```python
from build123d import *

# Parameters (mm, degrees)
F1_DEPTH = 50


with BuildPart() as f1:
    # F0 (on Right) → F1 (new body)
    with BuildSketch(Plane.YZ):
        with BuildLine():
            Line((-33.1, -0.25), (-33.35, -0.25))
            Line((-33.35, -0.25), (-33.35, 0))
            Line((-33.35, 0), (-33.35, 50.8))
            Line((-33.35, 50.8), (-33.35, 51.05))
            Line((-33.35, 51.05), (-33.1, 51.05))
            Line((-33.1, 51.05), (-31.35, 51.05))
            ThreePointArc((-31.35, 51.05), (-30.642893, 51.342893), (-30.35, 52.05))
            ThreePointArc((-30.35, 52.05), (-30.642893, 52.757107), (-31.35, 53.05))
            Line((-31.35, 53.05), (-33.1, 53.05))
            ThreePointArc((-33.1, 53.05), (-34.69099, 52.39099), (-35.35, 50.8))
            Line((-35.35, 50.8), (-35.35, 0))
            ThreePointArc((-35.35, 0), (-33.885534, -3.535534), (-30.35, -5))
            Line((-30.35, -5), (25.4, -5))
            ThreePointArc((25.4, -5), (28.935534, -3.535534), (30.4, 0))
            Line((30.4, 0), (30.4, 14))
            ThreePointArc((30.4, 14), (30.107107, 14.707107), (29.4, 15))
            ThreePointArc((29.4, 15), (28.692893, 14.707107), (28.4, 14))
            Line((28.4, 14), (28.4, 0))
            Line((28.4, 0), (28.4, -3))
            Line((28.4, -3), (25.4, -3))
            Line((25.4, -3), (0, -3))
            Line((0, -3), (-3, -3))
            Line((-3, -3), (-3, 0))
            Line((-3, 0), (-3, 48.35))
            ThreePointArc((-3, 48.35), (-4.376598, 51.673402), (-7.7, 53.05))
            Line((-7.7, 53.05), (-9.45, 53.05))
            ThreePointArc((-9.45, 53.05), (-10.157107, 52.757107), (-10.45, 52.05))
            ThreePointArc((-10.45, 52.05), (-10.157107, 51.342893), (-9.45, 51.05))
            Line((-9.45, 51.05), (-7.7, 51.05))
            Line((-7.7, 51.05), (-7.45, 51.05))
            Line((-7.45, 51.05), (-7.45, 50.8))
            Line((-7.45, 50.8), (-7.45, 0))
            Line((-7.45, 0), (-7.45, -0.25))
            Line((-7.45, -0.25), (-7.7, -0.25))
            Line((-7.7, -0.25), (-33.1, -0.25))
        make_face()
        with BuildLine():
            Line((-33.35, 51.05), (-33.35, 50.8))
            ThreePointArc((-33.35, 50.8), (-33.276777, 50.976777), (-33.1, 51.05))
            Line((-33.1, 51.05), (-33.35, 51.05))
        make_face()
        with BuildLine():
            ThreePointArc((-7.7, 51.05), (-7.523223, 50.976777), (-7.45, 50.8))
            Line((-7.45, 50.8), (-7.45, 51.05))
            Line((-7.45, 51.05), (-7.7, 51.05))
        make_face()
        with BuildLine():
            ThreePointArc((0, -3), (-2.12132, -2.12132), (-3, 0))
            Line((-3, 0), (-3, -3))
            Line((-3, -3), (0, -3))
        make_face()
        with BuildLine():
            ThreePointArc((-7.45, 0), (-7.523223, -0.176777), (-7.7, -0.25))
            Line((-7.7, -0.25), (-7.45, -0.25))
            Line((-7.45, -0.25), (-7.45, 0))
        make_face()
        with BuildLine():
            Line((-33.35, 0), (-33.35, -0.25))
            Line((-33.35, -0.25), (-33.1, -0.25))
            ThreePointArc((-33.1, -0.25), (-33.276777, -0.176777), (-33.35, 0))
        make_face()
        with BuildLine():
            ThreePointArc((28.4, 0), (27.52132, -2.12132), (25.4, -3))
            Line((25.4, -3), (28.4, -3))
            Line((28.4, -3), (28.4, 0))
        make_face()
    extrude(amount=-F1_DEPTH)


solid = f1.part
```
Work out the finished part from the listing and answer in its coordinate system (mm). A direction names the side the tool comes from. Give positions to 0.01 mm unless a question says otherwise; leave off trailing zeros. Order: outer loops, then holes, each group sorted by start corner. A loop starts at its lowest first (then second) coordinate and runs counter-clockwise, first axis right, second up. Notation, with made-up numbers: (85, 6) - (117, 6) arc R17 cw to (117, 14) - close; hole circle Ø11 at (-26.5, -5.5). An arc over 180 degrees is marked (long way). One line per item, written item: value. Start each with the question number.
1. Consider line 1 (Y direction, x = -16, z = 2.5); line 2 (Y direction, x = -24.5, z = 39.5); line 3 (Z direction, x = -16.5, y = 19.5). Determine where each line is inside the solid, lowest interval first.
2. Section A-A, the plane z = 19 is taken. Write down the section's boundary in (x, y).
3. Each of these flat-tipped pins is pushed along its axis until it touches: pin 1 Ø0.5 at (x, y) = (-29.5, -32) entering from -Z; pin 2 Ø4 at (x, y) = (-44.5, 12.5) entering from +Z; pin 3 Ø1.5 at (x, z) = (-20.5, 46) entering from +Y. Where does it stop, or does it pass through?
4. Which of the six approach directions +Z, -Z, +X, -X, +Y, -Y give full straight-line access (tool end or side, diameter ignored) to faces 1 (the face through (-50, -5, 16)), 2 (the face through (-25, 28.4, 7)), 3 (the face through (-25, -20, -0.25))?
5. For a pull along Y with two mould halves and no side action, classify faces 4 (the face through (-25, -32, 51.05)), 5 (the face through (-25, -35.35, 26)), 6 (the face through (-24.65, -4.34, 51.637)), 7 (the face through (-25, -9, 51.05)) as released by +Y, released by -Y, zero draft, split by the parting line, or undercut.
6. Section B-B, the plane z = 10 is taken. Write down the section's boundary in (x, y).
7. Section D-D, the plane y = -17 is taken. Write down the section's boundary in (x, z).
Filled sheet:
1. line 1: -35.35 to -33.35, -7.45 to -3, 28.4 to 30.4
1. line 2: -35.35 to -33.35, -7.45 to -3
1. line 3: -5 to -3
2. outline: (-50, -35.35) - (0, -35.35) - (0, -33.35) - (-50, -33.35) - close; (-50, -7.45) - (0, -7.45) - (0, -3) - (-50, -3) - close
3. pin 1: z = -4.8
3. pin 2: z = -3
3. pin 3: y = -3
4. face 1: +Z, -Z, -X, +Y, -Y
4. face 2: +Z, +X, -X
4. face 3: +X, -X
5. face 4: undercut
5. face 5: released by -Y
5. face 6: released by +Y
5. face 7: undercut
6. outline: (-50, -35.35) - (0, -35.35) - (0, -33.35) - (-50, -33.35) - close; (-50, -7.45) - (0, -7.45) - (0, -3) - (-50, -3) - close; (-50, 28.4) - (0, 28.4) - (0, 30.4) - (-50, 30.4) - close
7. outline: (-50, -5) - (0, -5) - (0, -0.25) - (-50, -0.25) - close
